Read the model definition and answer for the solid it produces. Units are mm, in the model's axes. A direction names the side the tool comes from. Coordinates: 2 decimals unless noted, no trailing zeros. Order: outer loops, then holes, each group sorted by start corner. A loop starts at its lowest first (then second) coordinate and runs counter-clockwise, first axis right, second up. Notation, with made-up numbers: (-22.75, -4.5) -> (7.25, -4.5) arc R15 ccw to (7.25, 22.5) -> close; hole circle Ø6 at (53, 54.25). An arc over 180 degrees is marked (long way). Answer as a JSON object with one key per item and string values. Group by question number.
1) Section C-C on x = -9.5 is taken. Determine the outline of the cut face in (y, z).
2) Section A-A on z = 0 is taken. Determine the outline of the cut face in (x, y), and give its area (3 significant figures).
3) Consider L1, parallel to Y at x = -18, z = -28; L2, parallel to X at y = 8.25, z = 0; L3, parallel to X at y = 6.25, z = -1. Determine where each line is inside the solid, lowest interval first.
4) Section D-D on z = 9.5 is taken. Determine the outline of the cut face in (x, y), and give its area (3 significant figures).
5) Given pin 1 (6 mm diameter, centred on y = 9, z = -16.5, fed in from +X); pin 2 (4 mm diameter, centred on x = -10, y = 6, fed in from +Z); pin 3 (11.5 mm diameter, centred on x = 0, z = 0, fed in from -Y); pin 4 (6 mm diameter, centred on x = -20, y = 8.5, fed in from +Z), each flat-ended and moving along its own axis, determine where each tip first touches the part or whether it passes through.
6) A tool of negligible diameter and unlimited length cuts with its end or side. For faces 4 (the flat face through (-21, 9, 26)), 5 (the cylindrical face through (-21, 10, -28)), from which of +Z, -Z, +X, -X, +Y, -Y can it reach the whole face along a straight path? Write none if from no direction.
7) Determine the mould class of faces 1 (the cylindrical face through (-21, 1, -28)), 2 (the cylindrical face through (-4.88, 5.92, -1.08)), 3 (the flat face through (-21, 3, 26)) for opening direction Z: released by +Z, released by -Z, zero draft, split by the parting line, or undercut.
8) Section B-B on x = 0 is taken. Determine the outline of the cut face in (y, z).
from build123d import *

# Parameters (mm, degrees)
SKETCH1_R           = 35
SKETCH1_R_2         = 5
BOSS_EXTRUDE1_DEPTH = 12
SKETCH2_W           = 1.873405934
SKETCH2_H           = 6


with BuildPart() as part:
    # Sketch1 → Boss-Extrude1 (new body)
    with BuildSketch(Plane(origin=(0, 0, 0), x_dir=(1, 0, 0), z_dir=(0, 1, 0))):
        with Locations(Location((0, 0, 0), (0, 0, 270))):
            Circle(SKETCH1_R)
        with Locations(Location((0, 0, 0), (0, 0, 270))):
            Circle(SKETCH1_R_2, mode=Mode.SUBTRACT)
    extrude(amount=BOSS_EXTRUDE1_DEPTH)

    # Sketch2 → Cut-Revolve1 (revolve, cut)
    with BuildSketch(Plane.XY, mode=Mode.PRIVATE) as cut_revolve1_sk:
        with Locations((-34.063297033, 6)):
            Rectangle(SKETCH2_W, SKETCH2_H)
    revolve(cut_revolve1_sk.sketch.rotate(Axis((0, 28.885066711, 0), (0, -1, 0)), 270), axis=Axis((0, 28.885066711, 0), (0, -1, 0)), mode=Mode.SUBTRACT)


solid = part.part
Worked answers:
{
 "1": {"outline": "(0, -33.69) -> (3, -33.69) -> (3, -31.74) -> (9, -31.74) -> (9, -33.69) -> (12, -33.69) -> (12, 33.69) -> (9, 33.69) -> (9, 31.74) -> (3, 31.74) -> (3, 33.69) -> (0, 33.69) -> close"},
 "2": {"outline": "(-35, 0) -> (-5, 0) -> (-5, 12) -> (-35, 12) -> (-35, 9) -> (-33.13, 9) -> (-33.13, 3) -> (-35, 3) -> close; (5, 0) -> (35, 0) -> (35, 3) -> (33.13, 3) -> (33.13, 9) -> (35, 9) -> (35, 12) -> (5, 12) -> close", "area": "698 mm²"},
 "3": {"L1": "y = 0 to 3, 9 to 12", "L2": "x = -33.13 to -5, 5 to 33.13", "L3": "x = -33.11 to -4.9, 4.9 to 33.11"},
 "4": {"outline": "(-33.69, 0) -> (33.69, 0) -> (33.69, 3) -> (31.74, 3) -> (31.74, 9) -> (33.69, 9) -> (33.69, 12) -> (-33.69, 12) -> (-33.69, 9) -> (-31.74, 9) -> (-31.74, 3) -> (-33.69, 3) -> close", "area": "785 mm²"},
 "5": {"pin 1": "stops at x = 32.29", "pin 2": "stops at z = 32.15", "pin 3": "stops at y = 0", "pin 4": "stops at z = 30.57"},
 "6": {"face 4": "none", "face 5": "+Y, -Y"},
 "7": {"face 1": "split by the parting line", "face 2": "undercut", "face 3": "zero draft"},
 "8": {"outline": "(0, -35) -> (3, -35) -> (3, -33.13) -> (9, -33.13) -> (9, -35) -> (12, -35) -> (12, -5) -> (0, -5) -> close; (0, 5) -> (12, 5) -> (12, 35) -> (9, 35) -> (9, 33.13) -> (3, 33.13) -> (3, 35) -> (0, 35) -> close"}
}
